Part model, mm, in its own coordinate system. A direction names the side the tool comes from. Give positions to 0.01 mm unless a question says otherwise; leave off trailing zeros. Order: outer loops, then holes, each group sorted by start corner. A loop starts at its lowest first (then second) coordinate and runs counter-clockwise, first axis right, second up.
1. Probe line 1 (Y direction, x = 2, z = 1.25); line 2 (Y direction, x = -1, z = 0.5); line 3 (Y direction, x = -1.5, z = -0.75). List the from-to ranges inside material, lowest first.
2. Slice it at A-A on z = 0. List the corners of the cut face in (x, y), and give its area (3 significant figures).
3. Mould opens along X. For faces 1 (the flat face through (0, -8, 0)), 2 (the cylindrical face through (1.25, 2.91, 0.02)), 3 (the conical face through (2.92, 3.38, -0.06)) say: +X half, -X half, draft (parallel to the pull), parting line (faces both ways), or undercut.
4. Slice it at B-B on x = 0. List the corners of the cut face in (y, z), and give its area (3 significant figures).
5. Drop flat-ended pins along their axis: pin 1 Ø1 at (x, z) = (-2, -2.5) entering from -Y; pin 2 Ø3.5 at (x, z) = (-1.5, 1) entering from -Y; pin 3 Ø1 at (x, z) = (0, 0.5) entering from +Y; pin 4 Ø4 at (y, z) = (-1.5, 2) entering from +X. Give the stop position or say it passes through.
6. Which spindle directions (+Z, -Z, +X, -X, +Y, -Y) get a long thin tool onto all of the face, cutting with end or side? Do faces 4 (the cylindrical face through (0, -5, -2)), 5 (the cylindrical face through (-1.25, 2.91, -0.02)), 6 (the flat face through (-0.6, 2, 0)), 7 (the flat face through (1, 0, -2)), 8 (the cylindrical face through (1.615, 1.42, 3.105)). Say none if no direction does.
7. Slice it at C-C on y = 2. List the corners of the cut face in (x, z).
Autodesk Inventor part; units mm, degrees
ref_plane "YZ Plane" through (0, 0, 0) normal (1, 0, 0) x (0, 1, 0)
ref_plane "XZ Plane" through (0, 0, 0) normal (0, 1, 0) x (-1, 0, 0)
ref_plane "XY Plane" through (0, 0, 0) normal (0, 0, 1) x (1, 0, 0)
sketch "Sketch1" plane through (0, 0, 0) normal (0, 0, 1) x (1, 0, 0)
  line L0 (3.5, 0) -> (3.5, 3.5)
  line L1 (3.5, 3.5) -> (0, 3.5)
  line L2 (3.5, 0) -> (1.4, 0)
  line L3 (1.4, 0) -> (1.4, -3)
  line L4 (1.4, -3) -> (2, -3)
  line L5 (2, -3) -> (2, -8)
  line L6 (2, -8) -> (0, -8)
  line L7 (0, 3.5) -> (0, -8)
  point P0 (0, 0)
  dimension "d0" = 7
  dimension "d2" = 2.8
  dimension "d3" = 4
  dimension "d4" = 3.5
  dimension "d5" = 5
  dimension "d6" = 8
revolve "Вращение1" add sketch "Sketch1" angle 360 about axis through (0, 3.5, 0) along (0, -1, 0)
sketch "Sketch2" plane through (0, 3.5, 0) normal (0, 1, 0) x (1, 0, 0)
  circle A0 centre (0, 0) radius 3.5 construction
  circle A1 centre (0, 0) radius 1.25
  dimension "d31" = 2.5
extrude "Выдавливание1" cut sketch "Sketch2" against normal blind 1.2
chamfer "Фаска1" distance 0.7 angle 45 1 edges at (-3.5, 3.5, 0)
sketch "Sketch3" plane through (0, 0, 0) normal (0, 0, 1) x (1, 0, 0)
  line L0 (0, 0) -> (0, 3.5)
  line L1 (-2.3552, 0) -> (2.3552, 0) construction
  line L2 (-3.5, 3.5) -> (3.5, 3.5) construction
  line L3 (-0.6, 3.5) -> (0.6, 3.5)
  line L4 (0.6, 3.5) -> (0.6, 0.8)
  line L5 (0.6, 0.8) -> (-0.6, 0.8)
  line L6 (-0.6, 0.8) -> (-0.6, 3.5)
  dimension "d8" = 0.8
  dimension "d9" = 1.2
extrude "Выдавливание2" cut sketch "Sketch3" along normal through all both and the other way through all
fillet "Сопряжение1" radius 0.2 2 edges at (-1.4, 0, 0) (-1.4, -3, 0)
thread "Резьба1"
chamfer "Фаска2" distance 0.7 angle 45 1 edges at (-2, -8, 0)
equation "\"d31\" = d3_"
equation "\"d32\" = h3"
equation "\"d21\" = C1"
equation "\"d8\" = h2"
equation "\"d9\" = n"
equation "\"d12\" = R"
equation "\"d13\" = b"
equation "\"d15\" = C1"
equation "\"d0\" = D"
equation "\"d2\" = d1"
equation "\"d3\" = d_"
equation "\"d4\" = k1"
equation "\"d5\" = b"
equation "\"d6\" = l_"
equation "\"D\" = 7"
equation "\"d_\" = 4"
equation "\"l_\" = 8"
equation "\"b\" = 5"
equation "\"d1\" = 2.8"
equation "\"R\" = 0.2"
equation "\"C1\" = 0.7"
equation "\"h2\" = 0.8"
equation "\"n\" = 1.2"
equation "\"h3\" = 1.2"
equation "\"k1\" = 3.5"
equation "\"d3_\" = 2.5"
equation "\"G\" = l_ - b"
properties part number "Винт 3 M4-6gx8 ГОСТ 10336-80" material "Сталь, мягкая"
Data:
1. line 1: y = 0 to 3.5
1. line 2: y = -8 to 2.3
1. line 3: y = -7.62 to -3, 0 to 3.5
2. outline: (-3.5, 0) - (-1.6, 0) arc R0.2 cw to (-1.4, -0.2) - (-1.4, -2.8) arc R0.2 cw to (-1.6, -3) - (-2, -3) - (-2, -7.3) - (-1.3, -8) - (1.3, -8) - (2, -7.3) - (2, -3) - (1.6, -3) arc R0.2 cw to (1.4, -2.8) - (1.4, -0.2) arc R0.2 cw to (1.6, 0) - (3.5, 0) - (3.5, 2.8) - (2.8, 3.5) - (1.25, 3.5) - (1.25, 2.3) - (0.6, 2.3) - (0.6, 0.8) - (-0.6, 0.8) - (-0.6, 2.3) - (-1.25, 2.3) - (-1.25, 3.5) - (-2.8, 3.5) - (-3.5, 2.8) - close
2. area: 47.2 mm2
3. face 1: draft
3. face 2: undercut
3. face 3: +X half
4. outline: (-8, -1.3) - (-7.3, -2) - (-3, -2) - (-3, -1.6) arc R0.2 cw to (-2.8, -1.4) - (-0.2, -1.4) arc R0.2 cw to (0, -1.6) - (0, -3.5) - (0.8, -3.5) - (0.8, 3.5) - (0, 3.5) - (0, 1.6) arc R0.2 cw to (-0.2, 1.4) - (-2.8, 1.4) arc R0.2 cw to (-3, 1.6) - (-3, 2) - (-7.3, 2) - (-8, 1.3) - close
4. area: 33.5 mm2
5. pin 1: stops at y = 0
5. pin 2: stops at y = -8
5. pin 3: stops at y = 0.8
5. pin 4: stops at x = 3.43
6. face 4: -Y
6. face 5: +Y
6. face 6: +Z, -Z, +Y
6. face 7: none
6. face 8: +Y, -Y
7. outline: (-0.6, -3.45) - (-0.6, 3.45) arc R3.5 ccw to start; (0.6, -3.45) arc R3.5 ccw to (0.6, 3.45) - close
